For this review, take the finished solid that the model builds, in its own axes (mm). A direction names the side the tool comes from. Coordinates: 2 decimals unless noted, no trailing zeros. Loops run counter-clockwise (first coordinate to the right, second up) from the corner with the lowest first, then second, coordinate; pieces in that order, holes last.
Autodesk Fusion 360 part; units mm, degrees
sketch "T-track" plane through (0, 0, 0) normal (1, 0, 0) x (0, 1, 0)
  line L0 (-15, 0) -> (15, 0)
  line L1 (15, 0) -> (15, 12.8)
  line L2 (-15, 12.8) -> (-15, 0)
  line L3 (9.65, 12.8) -> (9.65, 7.8)
  line L4 (-9.65, 7.8) -> (-9.65, 12.8)
  line L5 (-12, 7.8) -> (-12, 3)
  line L6 (-12, 3) -> (12, 3)
  line L7 (12, 3) -> (12, 7.8)
  line L8 (15, 12.8) -> (9.65, 12.8)
  line L9 (-9.65, 12.8) -> (-15, 12.8)
  line L10 (12, 7.8) -> (9.65, 7.8)
  line L11 (-9.65, 7.8) -> (-12, 7.8)
  dimension "d1" = 30
  dimension "d2" = 12.8
  dimension "d3" = 19.3
  dimension "d4" = 5
  dimension "d5" = 9.65
  dimension "d6" = 24
  dimension "d7" = 4.8
  dimension "d8" = 12
extrude "Extrude1" add sketch "T-track" along normal mid plane 500
sketch "Holes" plane through (0, 0, 3) normal (0, 0, 1) x (-1, 0, 0)
  line L0 (250, 12) -> (-250, 12)
  line L1 (-250, 12) -> (-250, -12)
  line L2 (-250, -12) -> (250, -12)
  line L3 (250, -12) -> (250, 12)
  line L4 (250, 0) -> (-250, 0) construction
  circle A0 centre (225, 0) radius 2
  circle A1 centre (-225, 0) radius 2
  circle A2 centre (-75, 0) radius 2
  circle A3 centre (75, 0) radius 2
  dimension "d12" = 4
  dimension "d13" = 4
  dimension "d14" = 25
  dimension "d22" = 4
  dimension "d23" = 4
  dimension "d24" = 150
  dimension "d25" = 150
  dimension "d26" = 150
  dimension "d27" = 25
extrude "Extrude2" cut sketch "Holes" against normal through all contours A0 | A1 | A2 | A3
chamfer "Chamfer2" distance 2 angle 45 4 edges at (226.8647, -0.7232, 3) (76.8647, -0.7232, 3) (-73.1353, -0.7232, 3) (-223.1353, -0.7232, 3)
equation "d5 = ( 19.3 / 2 ) * 1 mm"
equation "d8 = ( 24 / 2 ) * 1 mm"
equation "d12 = d13"
equation "d22 = d13"
equation "d23 = d13"
Q1. For pin 1 Ø5 at (y, z) = (9.5, 5.5) entering from +X; pin 2 Ø6.5 at (x, y) = (-225, 0) entering from +Z; pin 3 Ø5 at (x, y) = (225, 0) entering from +Z, all flat-tipped, find the tip position at first contact; note any pin that passes through.
Q2. The part is to be moulded in two halves that separate along Y. For faces 1 (the face through (-250, 0, 2)), 2 (the face through (-4, -15, 6)), 3 (the face through (77.123, -0.093, 1.125)), say which applies: +Y half, -Y half, draft (parallel to the pull), parting line (faces both ways), or undercut.
Q3. Machinability: for faces 4 (the face through (-4, 0, 0)), 5 (the face through (-4, 0, 3)), which of the approach directions +Z, -Z, +X, -X, +Y, -Y give a long, thin tool a straight path to every point of the face, cutting with its end or side? Answer none if there is none.
Q4. Wall thickness on probe 1 along X at (y, z) = (0, 0.85); probe 2 along Y at (x, z) = (75, 0.65); probe 3 along Z at (x, y) = (-193, 11.25): over which ranges is each line inside the solid? List them lowest first.
Q5. Consider section A-A (x = -189). State the section outline as (y, z) points, then the cut area to 3 significant figures.
Model answer:
1. pin 1: stops at x = 250
1. pin 2: stops at z = 2.25
1. pin 3: stops at z = 1.5
2. face 1: draft
2. face 2: -Y half
2. face 3: undercut
3. face 4: -Z, +X, -X, +Y, -Y
3. face 5: +X, -X
4. probe 1: x = -250 to -227, -223 to -77, -73 to 73, 77 to 223, 227 to 250
4. probe 2: y = -15 to -2, 2 to 15
4. probe 3: z = 0 to 3, 7.8 to 12.8
5. outline: (-15, 0) - (15, 0) - (15, 12.8) - (9.65, 12.8) - (9.65, 7.8) - (12, 7.8) - (12, 3) - (-12, 3) - (-12, 7.8) - (-9.65, 7.8) - (-9.65, 12.8) - (-15, 12.8) - close
5. area: 172 mm2
